Part model, mm, in its own coordinate system. A direction names the side the tool comes from. Give positions to 0.01 mm unless a question says otherwise; leave off trailing zeros. Order: outer loops, then holes, each group sorted by start corner. A loop starts at its lowest first (then second) coordinate and runs counter-clockwise, first axis right, second up.
1. Drop flat-ended pins along their axis: pin 1 Ø5 at (x, y) = (-110, -114.5) entering from -Z; pin 2 Ø1.5 at (y, z) = (205.5, 69.5) entering from -X; pin 3 Ø4 at (x, y) = (156.5, 224) entering from -Z. Give the stop position or say it passes through.
2. Which spindle directions (+Z, -Z, +X, -X, +Y, -Y) get a long thin tool onto all of the face, cutting with end or side? Do faces 4 (the cylindrical face through (-221.59, 375.13, 61.57)), 5 (the conical face through (-22.67, -217.55, -102.1)). Say none if no direction does.
3. Slice it at C-C on y = 116. List the corners of the cut face in (x, z) (1 decimal).
4. Slice it at B-B on z = 0. List the corners of the cut face in (x, y).
5. Slice it at D-D on y = -238. List the corners of the cut face in (x, z).
6. Probe line 1 (X direction, y = 288, z = 0); line 2 (Z direction, x = -119, y = -107); line 3 (X direction, y = -152.5, z = -11.5). List the from-to ranges inside material, lowest first.
7. Mould opens along X. For faces 1 (the cylindrical face through (212.635, 225.4, 88.163)), 2 (the flat face through (20, -351.953, -16)), 3 (the cylindrical face through (-228.38, 225.4, -10.05)) say: +X half, -X half, draft (parallel to the pull), parting line (faces both ways), or undercut.
8. Slice it at A-A on x = 0. List the corners of the cut face in (y, z).
from build123d import *

# Parameters (mm, degrees)
SKETCH7_R           = 230.1875
SKETCH7_R_2         = 228.6
BOSS_EXTRUDE1_DEPTH = 457.2
SKETCH9_R           = 10.795
CUT_EXTRUDE1_DEPTH  = 304.8


with BuildPart() as part:
    # Sketch7 → Boss-Extrude1 (new body)
    with BuildSketch(Plane(origin=(0, 0, 0), x_dir=(1, 0, 0), z_dir=(0, 1, 0))):
        Circle(SKETCH7_R)
        Circle(SKETCH7_R_2, mode=Mode.SUBTRACT)
    extrude(amount=BOSS_EXTRUDE1_DEPTH)

    # Sketch8 → Revolve1 (revolve)
    with BuildSketch(Plane.XY):
        Polygon((228.6, 0), (230.1875, 0), (26.9875, -351.952724098), (25.4, -351.952724098), align=None)
    revolve(axis=Axis((0, 0, 0), (0, -1, 0)))

    # Sketch9 → Cut-Extrude1 (cut)
    with BuildSketch(Plane(origin=(0, 0, 0), x_dir=(0, 0, -1), z_dir=(1, 0, 0))):
        with Locations((-57.15, 384.980800527)):
            Circle(SKETCH9_R)
    extrude(amount=-CUT_EXTRUDE1_DEPTH, mode=Mode.SUBTRACT)


solid = part.part
Data:
1. pin 1: stops at z = -124.68
1. pin 2: stops at x = -219.68
1. pin 3: stops at z = -170.63
2. face 4: -X
2. face 5: -Y
3. outline: circle Ø460.4 at (0, 0); hole circle Ø457.2 at (0, 0)
4. outline: (-230.19, 0) - (-26.99, -351.95) - (-25.4, -351.95) - (-228.6, 0) - (-228.6, 457.2) - (-230.19, 457.2) - close; (25.4, -351.95) - (26.99, -351.95) - (230.19, 0) - (230.19, 457.2) - (228.6, 457.2) - (228.6, 0) - close
5. outline: circle Ø185.56 at (0, 0); hole circle Ø182.38 at (0, 0)
6. line 1: x = -230.19 to -228.6, 228.6 to 230.19
6. line 2: z = -119.17 to -116.91, 116.91 to 119.17
6. line 3: x = -141.68 to -140.08, 140.08 to 141.68
7. face 1: parting line
7. face 2: draft
7. face 3: undercut
8. outline: (-351.95, -26.99) - (0, -230.19) - (457.2, -230.19) - (457.2, -228.6) - (0, -228.6) - (-351.95, -25.4) - close; (-351.95, 25.4) - (0, 228.6) - (457.2, 228.6) - (457.2, 230.19) - (0, 230.19) - (-351.95, 26.99) - close
